Model file for the job. Use its own axes, mm. Face numbers are marked on the shaded views. Coordinates: 2 decimals unless noted, no trailing zeros. Loops run counter-clockwise (first coordinate to the right, second up) from the corner with the lowest first, then second, coordinate; pieces in that order, holes last. Notation, with made-up numbers: (54, -38) -> (86, -38) arc R21 ccw to (86, -14) -> close; hole circle Ø7 at (70.25, 0.25). An arc over 180 degrees is marked (long way). Use one line per item in the form item = value.
```python
from build123d import *

# Parameters (mm, degrees)
F0_W     = 190.5
F0_H     = 31.75
F1_DEPTH = 12.7
F3_DEPTH = 25.4
F4_R     = 1.75
F5_DEPTH = 12.7
F6_W     = 113.973523
F6_H     = 19.05
F7_DEPTH = 6.35
F8_R     = 3.175


with BuildPart() as f1:
    # F0 (on Right) → F1 (new body)
    with BuildSketch(Plane.YZ):
        with Locations((95.25, 15.875)):
            Rectangle(F0_W, F0_H)
    extrude(amount=F1_DEPTH)

    # F2 (on face) → F3 (cut)
    with BuildSketch(Plane.YZ.offset(12.7)):
        Polygon((139.7, 31.75), (190.5, 0), (190.5, 31.75), align=None)
    extrude(amount=-F3_DEPTH, mode=Mode.SUBTRACT)

    # F4 (on face) → F5 (cut)
    with BuildSketch(Plane.XZ):
        with Locations((6.35, 6.35)):
            Circle(F4_R)
        with Locations((6.35, 25.4)):
            Circle(F4_R)
    extrude(amount=-F5_DEPTH, mode=Mode.SUBTRACT)

    # F6 (on face) → F7 (cut)
    with BuildSketch(Plane(origin=(0, 0, 0), x_dir=(0, -1, 0), z_dir=(-1, 0, 0))):
        with Locations((-76.036761, 15.875)):
            Rectangle(F6_W, F6_H)
    extrude(amount=-F7_DEPTH, mode=Mode.SUBTRACT)

    # F8
    f8_edges = [f1.edges().sort_by_distance(p)[0] for p in [
        (3.175, 133.023523, 25.4),
        (3.175, 19.05, 25.4),
        (3.175, 19.05, 6.35),
        (3.175, 133.023523, 6.35),
    ]]
    fillet(f8_edges, radius=F8_R)


solid = f1.part
```
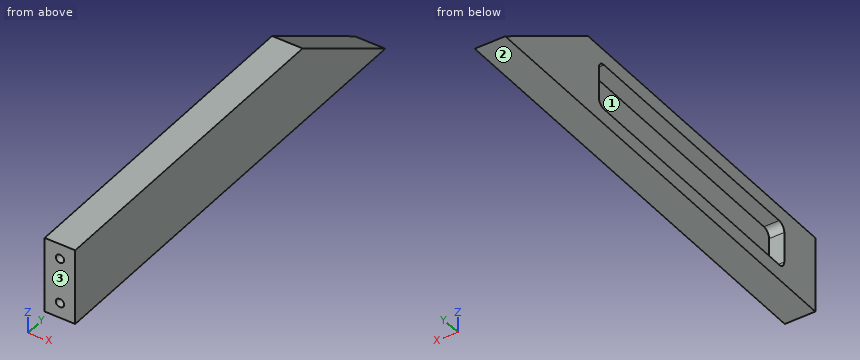
Q1. Mould opens along Z. For the marked faces 1, 2 and 3 say: released by +Z, released by -Z, zero draft, split by the parting line, or undercut.
Result:
face_1 = undercut
face_2 = released by -Z
face_3 = zero draft
Q2. Pin check, flat tips, straight feed: pin 1 Ø6 at (x, z) = (8.5, 9) entering from +Y; pin 2 Ø3 at (x, z) = (11.5, 12) entering from +Y; pin 3 Ø2 at (x, z) = (6.35, 6.35) entering from -Y. Stop position of each tip, or through.
Result:
pin_1 = 180.9
pin_2 = 173.7
pin_3 = 12.7
Q3. Band-saw the part on A-A, the plane y = 116.5. Write the cut outline in (x, z).
Result:
outline = (0, 0) -> (12.7, 0) -> (12.7, 31.75) -> (0, 31.75) -> (0, 25.4) -> (6.35, 25.4) -> (6.35, 6.35) -> (0, 6.35) -> close
Q4. Band-saw the part on D-D, the plane z = 2.5. Write the cut outline in (x, y), and give its area (3 significant figures).
Result:
outline = (0, 0) -> (12.7, 0) -> (12.7, 186.5) -> (0, 186.5) -> close
area = 2,370 mm2
Q5. Band-saw the part on B-B, the plane z = 20.5. Write the cut outline in (x, y), and give its area (3 significant figures).
Result:
outline = (0, 0) -> (12.7, 0) -> (12.7, 157.7) -> (0, 157.7) -> (0, 133.02) -> (6.35, 133.02) -> (6.35, 19.05) -> (0, 19.05) -> close
area = 1,280 mm2
Q6. Wall check: line 1 along Z through (x, y) = (6.35, 8.25); line 2 along X through (y, z) = (3, 6); line 3 along X through (y, z) = (47.5, 16). Give the ranges that are in metal, low to high.
Result:
line_1 = 0 to 4.6, 8.1 to 23.65, 27.15 to 31.75
line_2 = 0 to 4.64, 8.06 to 12.7
line_3 = 6.35 to 12.7
Q7. Band-saw the part on C-C, the plane x = 9.75. Write the cut outline in (y, z), and give its area (3 significant figures).
Result:
outline = (0, 0) -> (190.5, 0) -> (139.7, 31.75) -> (0, 31.75) -> close
area = 5,240 mm2
